from build123d import *

# Parameters (mm, degrees)
SKETCH1_W           = 15
SKETCH1_H           = 35
BOSS_EXTRUDE1_DEPTH = 5
SKETCH4_W           = 15
SKETCH4_H           = 1.5
CUT_EXTRUDE1_DEPTH  = 30
FILLET1_R           = 1
FILLET2_R           = 1
FILLET3_R           = 0.5
FILLET4_R           = 0.5
SKETCH5_W           = 15
SKETCH5_H           = 2
BOSS_EXTRUDE2_DEPTH = 1.5
SKETCH8_W           = 2
SKETCH8_H           = 0.5
CUT_EXTRUDE3_DEPTH  = 15
FILLET5_R           = 0.5


with BuildPart() as part:
    # Sketch1 → Boss-Extrude1 (new body)
    with BuildSketch(Plane(origin=(0, 0, 0), x_dir=(1, 0, 0), z_dir=(0, 1, 0))):
        Rectangle(SKETCH1_W, SKETCH1_H)
    extrude(amount=BOSS_EXTRUDE1_DEPTH)

    # Sketch4 → Cut-Extrude1 (cut)
    with BuildSketch(Plane.XY.offset(17.5)):
        with Locations((0, 2.5)):
            Rectangle(SKETCH4_W, SKETCH4_H)
    extrude(amount=-CUT_EXTRUDE1_DEPTH, mode=Mode.SUBTRACT)

    # Fillet1
    fillet1_edges = [part.edges().sort_by_distance(p)[0] for p in [
        (-7.5, 5, 0),
        (0, 5, 17.5),
        (7.5, 5, 0),
        (0, 5, -17.5),
    ]]
    fillet(fillet1_edges, radius=FILLET1_R)

    # Fillet2
    fillet2_edges = [part.edges().sort_by_distance(p)[0] for p in [
        (0, 0, 17.5),
        (-7.5, 0, 0),
        (0, 0, -17.5),
        (7.5, 0, 0),
    ]]
    fillet(fillet2_edges, radius=FILLET2_R)

    # Fillet3
    fillet3_edges = [part.edges().sort_by_distance(p)[0] for p in [
        (0, 3.25, -12.5),
    ]]
    fillet(fillet3_edges, radius=FILLET3_R)

    # Fillet4
    fillet4_edges = [part.edges().sort_by_distance(p)[0] for p in [
        (0, 1.75, -12.5),
    ]]
    fillet(fillet4_edges, radius=FILLET4_R)

    # Sketch5 → Boss-Extrude2 (add)
    with BuildSketch(Plane(origin=(0, 1.75, 0), x_dir=(1, 0, 0), z_dir=(0, 1, 0))):
        with Locations((0, -16.5)):
            Rectangle(SKETCH5_W, SKETCH5_H)
    extrude(amount=BOSS_EXTRUDE2_DEPTH)

    # Sketch8 → Cut-Extrude3 (cut)
    with BuildSketch(Plane(origin=(7.5, 0, 0), x_dir=(0, 0, -1), z_dir=(1, 0, 0))):
        with Locations((-16.5, 3)):
            Rectangle(SKETCH8_W, SKETCH8_H)
    extrude(amount=-CUT_EXTRUDE3_DEPTH, mode=Mode.SUBTRACT)

    # Fillet5
    fillet5_edges = [part.edges().sort_by_distance(p)[0] for p in [
        (-7.5, 2.75, 16.5),
        (0, 2.75, 15.5),
        (0, 2.75, 17.5),
        (7.5, 2.75, 16.5),
    ]]
    fillet(fillet5_edges, radius=FILLET5_R)


solid = part.part
Verification items for the finished model (mm, model axes). A direction names the side the tool comes from. Coordinates: 2 decimals unless noted, no trailing zeros. Order: outer loops, then holes, each group sorted by start corner. A loop starts at its lowest first (then second) coordinate and runs counter-clockwise, first axis right, second up.
Item 1: Section check B-B, the plane x = 5. Enter the section's corners in (y, z).
Filled in:
outline: (0, -16.5) arc R1 ccw to (1, -17.5) - (4, -17.5) arc R1 ccw to (5, -16.5) - (5, 16.5) arc R1 ccw to (4, 17.5) - (3.25, 17.5) - (3.25, -12) arc R0.5 cw to (2.75, -12.5) - (2.25, -12.5) arc R0.5 cw to (1.75, -12) - (1.75, 15.5) - (2.25, 15.5) arc R0.5 ccw to (2.75, 16) - (2.75, 17) arc R0.5 ccw to (2.25, 17.5) - (1, 17.5) arc R1 ccw to (0, 16.5) - close
Item 2: Section check A-A, the plane z = 0. Enter the section's corners in (x, y), then the cut area to 3 significant figures.
Filled in:
outline: (-7.5, 1) arc R1 ccw to (-6.5, 0) - (6.5, 0) arc R1 ccw to (7.5, 1) - (7.5, 1.75) - (-7.5, 1.75) - close; (-7.5, 3.25) - (7.5, 3.25) - (7.5, 4) arc R1 ccw to (6.5, 5) - (-6.5, 5) arc R1 ccw to (-7.5, 4) - close
area: 51.6 mm2
Item 3: Material ranges on L1, parallel to Y at x = -2.25, z = 0.5; L2, parallel to Z at x = -1.75, y = 4.1; L3, parallel to Z at x = -0.25, y = 2.1, recorded low to high.
Filled in:
L1: y = 0 to 1.75, 3.25 to 5
L2: z = -17.49 to 17.49
L3: z = -17.5 to -12.48, 15.5 to 17.5
Item 4: Release check for a two-part mould opening along Z. For faces 3 (the face through (0.1, 2.75, 16.5)), 4 (the face through (0, 1.75, 2)), 5 (the face through (0.105, 0.301, -17.215)) record: +Z half, -Z half, draft (parallel to the pull), parting line (faces both ways), or undercut.
Filled in:
face 3: draft
face 4: undercut
face 5: -Z half
Item 5: Access from +Z, -Z, +X, -X, +Y, -Y to the whole of each face (thin tool, end or side, straight path). Record for faces 1 (the face through (-7.215, 0.301, -0.245)), 2 (the face through (0, 3.25, 3)).
Filled in:
face 1: +Z, -Z, -X, -Y
face 2: +Z, +X, -X
